The figure shows three views and two pictorial views of one solid part (mm, origin at its lowest corner). Answer the questions. Coordinates: 2 decimals unless noted, no trailing zeros. Write each loop counter-clockwise with the first axis right and the second up, starting at its lowest first coordinate (ties: lowest second). Pieces come first, ordered by that corner, then holes.
Item 1: Section A-A (z = 10.5) is taken. Give the vertices of the cut face in (x, y), then the cut area to 3 significant figures.
Item 2: Section B-B (y = 44.5) is taken. Give the vertices of the cut face in (x, z).
Item 3: Section C-C (x = 80) is taken. Give the vertices of the cut face in (y, z).
Item 4: Each of these flat-tipped pins is pushed along its axis until it touches: P1, Ø4, axis at x = 692, z = 6, coming from the -Y side; P2, Ø6.5, axis at x = 3.5, z = 4, coming from the +Y side; P3, Ø4, axis at y = 62.5, z = 6, coming from the +X side; P4, Ø3, axis at x = 493, y = 27.5, coming from the -Z side. Where does it stop, or does it pass through?
Item 5: Section D-D (y = 7) is taken. Give the vertices of the cut face in (x, z).
Item 6: Straight lines are drawn through the part: probe 1 along Z at (x, y) = (612, 40); probe 2 along X at (y, z) = (6, 1.5); probe 3 along X at (y, z) = (84, 6). For each, find the intervals that lie inside material, in ascending order.
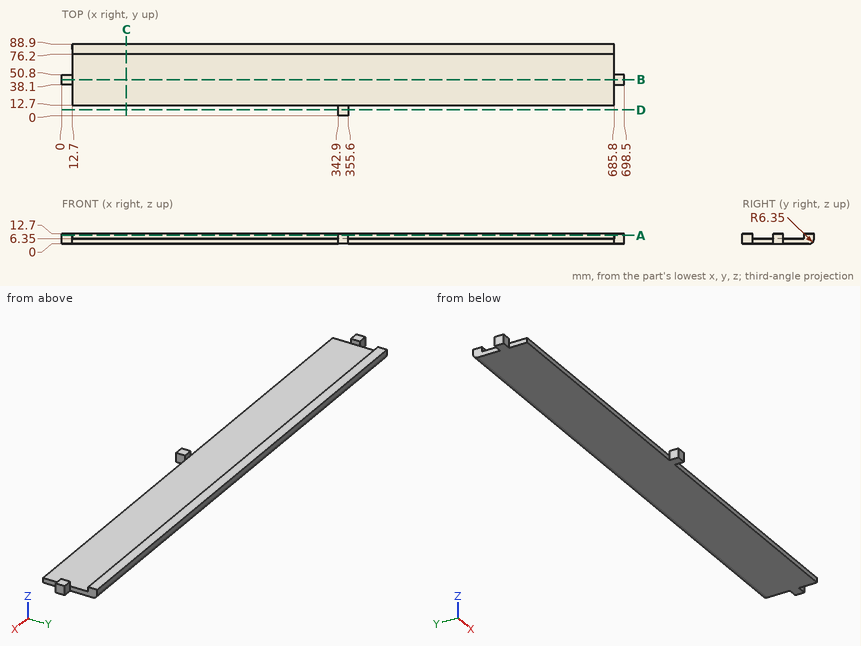
Established:
1. outline: (0, 38.1) - (12.7, 38.1) - (12.7, 50.8) - (0, 50.8) - close; (12.7, 76.2) - (685.8, 76.2) - (685.8, 88.9) - (12.7, 88.9) - close; (342.9, 0) - (355.6, 0) - (355.6, 12.7) - (342.9, 12.7) - close; (685.8, 38.1) - (698.5, 38.1) - (698.5, 50.8) - (685.8, 50.8) - close
1. area: 9,030 mm2
2. outline: (0, 0) - (698.5, 0) - (698.5, 12.7) - (685.8, 12.7) - (685.8, 6.35) - (12.7, 6.35) - (12.7, 12.7) - (0, 12.7) - close
3. outline: (12.7, 0) - (82.55, 0) arc R6.35 ccw to (88.9, 6.35) - (88.9, 12.7) - (76.2, 12.7) - (76.2, 6.35) - (12.7, 6.35) - close
4. P1: stops at y = 38.1
4. P2: stops at y = 50.8
4. P3: stops at x = 685.8
4. P4: stops at z = 0
5. outline: (342.9, 0) - (355.6, 0) - (355.6, 12.7) - (342.9, 12.7) - close
6. probe 1: z = 0 to 6.35
6. probe 2: x = 342.9 to 355.6
6. probe 3: x = 12.7 to 685.8
